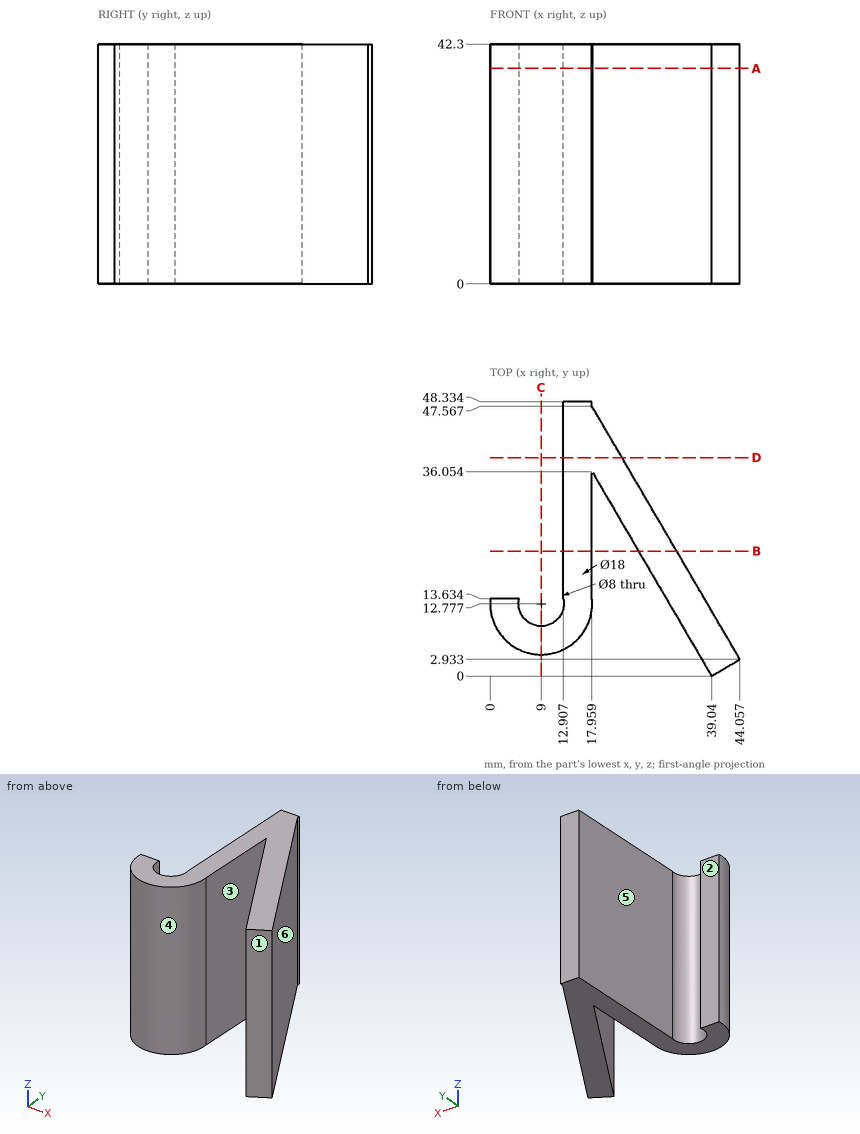
Could you check a few things on this drawing? It's one solid part, dimensions in mm from its lowest x, y, z. A direction names the side the tool comes from. Give positions to 0.01 mm unless a question says otherwise; leave off trailing zeros. Loops run counter-clockwise (first coordinate to the right, second up) from the corner with the lowest first, then second, coordinate; pieces in that order, holes last. Notation, with made-up numbers: M 24.5,-28 L 57.5,-28 A20 cw 57.5,-3 Z; hole C -36,51 d6. An arc over 180 degrees is marked long. One line per question, with ' | ' between items. Start each with the question number.
Q1. If we section it at A-A (z = 38): Please give me the cut outline in (x, y) (1 decimal).
Q2. If we section it at B-B (y = 22): Please give me the cut outline in (x, z).
Q3. If we mould it in two halves opening along X, with no side actions, what happens to the marked faces 3, 4, 5 and 6? For each: +X half, -X half, draft (parallel to the pull), parting line (faces both ways), or undercut.
Q4. For pin 1 Ø5 at (y, z) = (36, 12) entering from -X; pin 2 Ø6.5 at (y, z) = (28.5, 13) entering from +X; pin 3 Ø1.5 at (y, z) = (32.5, 23) entering from +X, each with a flat end and sliding along its axis, tell me the tip position at first contact or that it passes through.
Q5. If we section it at D-D (y = 38.5): Please give me the cut outline in (x, z).
Q6. For the marked faces 1 and 2, which set-ups out of +Z, -Z, +X, -X, +Y, -Y let a thin tool reach every point of the face, with its end or its side?
Q7. If I drill on line 1 (X direction, y = 12, z = 11.5) (1 decimal); line 2 (X direction, y = 22, z = 29) (1 decimal); line 3 (X direction, y = 14.5, z = 10) (1 decimal), over which ranges is the centre line in solid material (lowest first)? Write a range as from..to.
Q8. If we section it at C-C (x = 9): Please give me the cut outline in (y, z).
Computed:
1) outline: M 0,13.6 A9 ccw long 18,13.6 L 18,36.1 L 39,0 L 44.1,2.9 L 18,47.6 L 18,48.3 L 12.9,48.3 L 12.9,13.6 A4 cw long 5.1,13.6 Z
2) outline: M 12.91,0 L 17.96,0 L 17.96,42.3 L 12.91,42.3 Z; M 26.18,0 L 32.91,0 L 32.91,42.3 L 26.18,42.3 Z
3) face 3: undercut | face 4: undercut | face 5: -X half | face 6: +X half
4) pin 1: stops at x = 12.91 | pin 2: stops at x = 31.01 | pin 3: stops at x = 27.21
5) outline: M 12.91,0 L 23.26,0 L 23.26,42.3 L 12.91,42.3 Z
6) face 1: +Z, -Z, +X, -Y | face 2: +Z, -Z, -X, +Y
7) line 1: x = 0..5.1, 12.9..18, 32..38.8 | line 2: x = 12.9..18, 26.2..32.9 | line 3: x = 12.9..18, 30.6..37.3
8) outline: M 3.78,0 L 8.78,0 L 8.78,42.3 L 3.78,42.3 Z
